The model under review builds one solid part; all positions refer to its coordinate system, in mm. A direction names the side the tool comes from. Coordinates: 2 decimals unless noted, no trailing zeros. Order: outer loops, then holes, each group sorted by start corner. A loop starts at its lowest first (then second) coordinate and runs counter-clockwise, first axis right, second up. Notation, with made-up numbers: (-31.5, -9.75) -> (27.5, -9.75) arc R12 ccw to (27.5, 10.25) -> close; hole circle Ø3 at (42, 72.25). An arc over 180 degrees is marked (long way). Put each result on its own line as item: value.
from build123d import *

# Parameters (mm, degrees)
F0_W     = 50
F0_H     = 50
F0_W_2   = 48
F0_H_2   = 48
F1_DEPTH = 25
F2_DEPTH = 24


with BuildPart() as f1:
    # F0 (on Front) → F1 (new body, symmetric)
    with BuildSketch(Plane.XZ):
        Rectangle(F0_W, F0_H)
        Rectangle(F0_W_2, F0_H_2, mode=Mode.SUBTRACT)
        Rectangle(F0_W_2, F0_H_2)
    extrude(amount=F1_DEPTH, both=True)


with BuildPart() as f2:
    # F0 (on Front) → F2 (new body, symmetric)
    with BuildSketch(Plane.XZ):
        Rectangle(F0_W_2, F0_H_2)
    extrude(amount=F2_DEPTH, both=True)


with BuildPart() as f1_1:
    add(f1.part)

    # F3: cut F2
    add(f2.part, mode=Mode.SUBTRACT)


solid = f1_1.part
Item 1: Consider section A-A on x = -7.5. Write out the cut boundary in (y, z), and give its area (3 significant figures).
Answers below:
outline: (-25, -25) -> (25, -25) -> (25, 25) -> (-25, 25) -> close; hole (-24, -24) -> (24, -24) -> (24, 24) -> (-24, 24) -> close
area: 196 mm^2
Item 2: For faces 5 (the flat face through (-25, 0, 0)), 6 (the flat face through (0, 24, 0)), list the 3-axis set-ups (+Z, -Z, +X, -X, +Y, -Y) from which the entire face can be reached by the end or side of a thin tool; tool diameter is ignored.
Answers below:
face 5: +Z, -Z, -X, +Y, -Y
face 6: none
Item 3: For line 1 (X direction, y = -6.5, z = -1.5), list the stretches that pass through material, from the lowest coordinate up. Write a range as from..to.
Answers below:
line 1: -25..-24, 24..25
Item 4: Mouldability with a two-part tool opening along X and no side actions: class faces 1 (the flat face through (25, 0, 0)), 2 (the flat face through (0, 0, -24)), 3 (the flat face through (0, 0, 25)), 4 (the flat face through (0, -24, 0)) as +X half, -X half, draft (parallel to the pull), parting line (faces both ways), or undercut.
Answers below:
face 1: +X half
face 2: undercut
face 3: draft
face 4: undercut
